Design review of the part built by this model. Coordinates are the model's own, in mm. Face numbers are marked on the shaded views. A direction names the side the tool comes from. Coordinates: 2 decimals unless noted, no trailing zeros. Order: outer loops, then holes, each group sorted by start corner. A loop starts at its lowest first (then second) coordinate and runs counter-clockwise, first axis right, second up. Notation, with made-up numbers: M 62.25,18.25 L 80.25,18.25 A17 ccw 80.25,27.25 Z; hole C -17,87 d10. An arc over 180 degrees is marked long. Answer as a JSON object with one key per item and string values.
from build123d import *

# Parameters (mm, degrees)
ESQUISSE1_W             = 3.17
ESQUISSE1_H             = 11.950083308
BOSS_EXTRU_1_DEPTH      = 10
ESQUISSE3_R             = 4.5
ENL_V_MAT_EXTRU_1_DEPTH = 6.25
ESQUISSE4_R             = 4.5
ENL_V_MAT_EXTRU_2_DEPTH = 10
ENL_V_MAT_EXTRU_4_DEPTH = 10
BOSS_EXTRU_3_DEPTH      = 10
BOSS_EXTRU_4_DEPTH      = 10


with BuildPart() as part:
    # Esquisse1 → Boss.-Extru.1 (new body)
    with BuildSketch(Plane.XY):
        with Locations((1.585, 5.975041654)):
            Rectangle(ESQUISSE1_W, ESQUISSE1_H)
        with BuildLine():
            ThreePointArc((0, 0), (-18.018658069, 5.975041654), (0, 11.950083308))
            Line((0, 11.950083308), (0, 0))
        make_face()
        with BuildLine():
            ThreePointArc((3.17, 11.950083308), (8.623303343, 5.975041654), (3.17, 0))
            Line((3.17, 0), (3.17, 11.950083308))
        make_face()
    extrude(amount=BOSS_EXTRU_1_DEPTH)

    # Esquisse3 → Enlèv. mat.-Extru.1 (cut)
    with BuildSketch(Plane.XY):
        with Locations((8.623303343, 5.975041654)):
            Circle(ESQUISSE3_R)
        Polygon((-4.326089499, -0.75758567), (-0.341747487, 5.806586179), (-4.034316058, 12.539213503), (-11.71122664, 12.707668978), (-15.695568652, 6.143497129), (-12.003000081, -0.589130195), align=None)
    extrude(amount=ENL_V_MAT_EXTRU_1_DEPTH, mode=Mode.SUBTRACT)

    # Esquisse4 → Enlèv. mat.-Extru.2 (cut)
    with BuildSketch(Plane(origin=(0, 0, 6.25), x_dir=(-1, 0, 0), z_dir=(0, 0, -1))):
        with Locations((8.141028583, 5.951350622)):
            Circle(ESQUISSE4_R)
    extrude(amount=-ENL_V_MAT_EXTRU_2_DEPTH, mode=Mode.SUBTRACT)

    # Esquisse6 → Enlèv. mat.-Extru.4 (cut)
    with BuildSketch(Plane(origin=(0, 0, 6.25), x_dir=(-1, 0, 0), z_dir=(0, 0, -1))):
        with BuildLine():
            ThreePointArc((-6.935803343, 1.803430005), (-8.623303343, 5.975041654), (-6.935803343, 10.146653303))
            ThreePointArc((-6.935803343, 10.146653303), (-4.123303343, 5.975041654), (-6.935803343, 1.803430005))
        make_face()
    extrude(amount=-ENL_V_MAT_EXTRU_4_DEPTH, mode=Mode.SUBTRACT)

    # Esquisse7 → Boss.-Extru.3 (add)
    with BuildSketch(Plane(origin=(0, 0, 0), x_dir=(-1, 0, 0), z_dir=(0, 0, -1))):
        with BuildLine():
            ThreePointArc((-3.17, 0), (-7.646039968, -1.391747442), (-11.795192237, 0.789176718))
            ThreePointArc((-11.795192237, 0.789176718), (-9.270284793, 0.840128378), (-6.935803343, 1.803430005))
            ThreePointArc((-6.935803343, 1.803430005), (-5.214835319, 0.563575862), (-3.17, 0))
        make_face()
    extrude(amount=-BOSS_EXTRU_3_DEPTH)

    # Esquisse8 → Boss.-Extru.4 (add)
    with BuildSketch(Plane(origin=(0, 0, 0), x_dir=(-1, 0, 0), z_dir=(0, 0, -1))):
        with BuildLine():
            ThreePointArc((-3.17, 11.950083308), (-7.281636762, 12.926912072), (-10.879725241, 10.71026808))
            ThreePointArc((-10.879725241, 10.71026808), (-8.857814072, 10.77798979), (-6.935803343, 10.146653303))
            ThreePointArc((-6.935803343, 10.146653303), (-5.214835319, 11.386507446), (-3.17, 11.950083308))
        make_face()
    extrude(amount=-BOSS_EXTRU_4_DEPTH)


solid = part.part
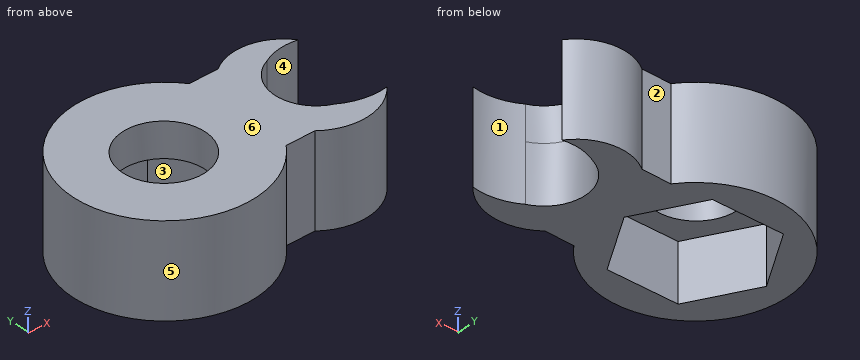
1) Mouldability with a two-part tool opening along Y and no side actions: class the marked faces 4, 5 and 6 as released by +Y, released by -Y, zero draft, split by the parting line, or undercut.
Taken from the geometry:
{"face 4": "undercut", "face 5": "split by the parting line", "face 6": "zero draft"}
2) Add section B-B (x = 6). State the section outline as (y, z) points.
Taken from the geometry:
{"outline": "M -1.32,0 L 2.32,0 L 2.32,10 L -1.32,10 Z; M 9.63,0 L 12.98,0 L 12.98,10 L 9.63,10 Z"}
3) Add section A-A (z = 2.25). State the section outline as (x, y) points.
Taken from the geometry:
{"outline": "M 0,0 L 3.17,0 A6.12 ccw 11.8,0.79 A6.84 cw 6.94,1.8 A4.5 cw 6.94,10.15 A5.8 cw 10.88,10.71 A5.52 ccw 3.17,11.95 L 0,11.95 A10 ccw long Z; hole M -15.7,6.14 L -12,-0.59 L -4.33,-0.76 L -0.34,5.81 L -4.03,12.54 L -11.71,12.71 Z"}
4) To check wall thickness, follow L1, parallel to Y at x = 5, z = 7.75; L2, parallel to X at y = 12.25, z = 8.5; L3, parallel to Y at x = 5.25, z = 7.75. State the ranges of each line that lie inside material, in increasing order.
Taken from the geometry:
{"L1": "y = -1.05 to 3.31, 8.64 to 12.82", "L2": "x = -15.8 to -0.23, 3.63 to 9.18", "L3": "y = -1.13 to 3, 8.95 to 12.87"}
5) Add section D-D (x = -11). State the section outline as (y, z) points.
Taken from the geometry:
{"outline": "M -3.57,0 L -0.61,0 L -0.61,6.25 L 2.48,6.25 L 2.48,10 L -3.57,10 Z; M 9.43,6.25 L 12.69,6.25 L 12.69,0 L 15.52,0 L 15.52,10 L 9.43,10 Z"}
6) Tool access review of the marked faces 1, 2 and 3: name each direction out of +Z, -Z, +X, -X, +Y, -Y from which nothing blocks a thin tool from reaching the whole face with its end or side.
Taken from the geometry:
{"face 1": "+Z, -Z", "face 2": "+Z, -Z, +Y", "face 3": "-Z"}
7) Add section C-C (y = 4.75). State the section outline as (x, z) points, and give its area (3 significant figures).
Taken from the geometry:
{"outline": "M -17.94,0 L -14.93,0 L -14.93,6.25 L -12.48,6.25 L -12.48,10 L -17.94,10 Z; M -3.8,6.25 L -0.98,6.25 L -0.98,0 L 4.29,0 L 4.29,10 L -3.8,10 Z", "area": "103 mm2"}
8) Insertion check: pin 1 Ø2.5 at (x, z) = (2, 4.5) entering from +Y; pin 2 Ø10 at (x, y) = (-5.5, 8) entering from -Z; pin 3 Ø5 at (y, z) = (10, 3) entering from -X; pin 4 Ø1 at (y, z) = (-1.5, 3) entering from -X. Each pin has a flat end and moves straight along its axis. Give the tip position at first contact, or say it passes through.
Taken from the geometry:
{"pin 1": "stops at y = 12.01", "pin 2": "stops at z = 0", "pin 3": "stops at x = -17.9", "pin 4": "stops at x = -15.18"}
